For this review, take the finished solid that the model builds, in its own axes (mm). A direction names the side the tool comes from. Give positions to 0.01 mm unless a question says otherwise; leave off trailing zeros. Loops run counter-clockwise (first coordinate to the right, second up) from the corner with the lowest first, then second, coordinate; pieces in that order, holes last. Notation, with made-up numbers: (11, -9.75) - (17, -9.75) arc R19 ccw to (17, 15.25) - close; hole circle Ø3 at (-5, 30). An arc over 180 degrees is marked (long way). Use CSV: the item, a comma, the result in double quotes. Start each with the question number.
1. Wall thickness on line 1 (Z direction, x = -20, y = 57); line 2 (X direction, y = 56, z = -103); line 3 (Y direction, x = -9, z = -40): over which ranges is each line inside the solid? List them lowest first.
2. Mouldability with a two-part tool opening along Y and no side actions: class faces 1 (the flat face through (-20, 10, -22)), 2 (the cylindrical face through (-9.86, 99.915, -38.698)), 3 (the cylindrical face through (-34.93, 63.007, -39.406)), 4 (the flat face through (-20, 20, -40)) as pulls with the +Y half, pulls with the -Y half, needs draft (parallel to the pull), parting line crosses it, or undercut.
3. For faces 5 (the flat face through (-20, 54, -93)), 6 (the flat face through (-20, 10, -58)), 7 (the flat face through (-20, 82, -48)), 8 (the flat face through (-20, 64, -94)), list the 3-axis set-ups (+Z, -Z, +X, -X, +Y, -Y) from which the entire face can be reached by the end or side of a thin tool; tool diameter is ignored.
4. Take a section at D-D on z = -101.5. Give the boundary of the cut face in (x, y).
5. Take a section at B-B on z = -40. Give the boundary of the cut face in (x, y).
6. For pin 1 (11 mm diameter, centred on y = 61.5, z = 11.5, fed in from +X); pin 2 (22 mm diameter, centred on x = -27.5, y = 8.5, fed in from -Z); pin 3 (3 mm diameter, centred on x = -23.5, y = 87, fed in from +Z) (3 decimals); pin 4 (6 mm diameter, centred on x = -20, z = 23, fed in from +Y) (3 decimals), all flat-tipped, find the tip position at first contact; note any pin that passes through.
7. Take a section at A-A on y = 7.5. Give the boundary of the cut face in (x, z).
8. Take a section at C-C on x = -7. Give the boundary of the cut face in (y, z).
Autodesk Inventor part; units mm, degrees
ref_plane "YZ Plane" through (0, 0, 0) normal (1, 0, 0) x (0, 1, 0)
ref_plane "XZ Plane" through (0, 0, 0) normal (0, 1, 0) x (-1, 0, 0)
ref_plane "XY Plane" through (0, 0, 0) normal (0, 0, 1) x (1, 0, 0)
sketch "Sketch1" plane through (0, 0, 0) normal (1, 0, 0) x (0, 1, 0)
  line L0 (0, 0) -> (54, 0)
  line L1 (54, 0) -> (54, -80)
  line L2 (54, -80) -> (0, -80)
  line L3 (0, -80) -> (0, 0)
  dimension "d0" = 80
  dimension "d1" = 54
extrude "Extrusion1" add sketch "Sketch1" against normal blind 40
sketch "Sketch2" plane through (0, 0, 0) normal (1, 0, 0) x (0, 0, -1)
  line L0 (22, 20) -> (58, 20)
  line L1 (0, 0) -> (80, 0)
  line L2 (0, 54) -> (80, 54)
  line L3 (40, 54) -> (40, 0)
  line L4 (22, 20) -> (22, 0)
  line L5 (58, 20) -> (58, 0)
  line L6 (22, 0) -> (58, 0)
  line L7 (80, 0) -> (0, 0)
  point P0 (40, 20)
  dimension "d4" = 36
  dimension "d5" = 20
extrude "Extrusion2" cut sketch "Sketch2" against normal blind 40
sketch "Sketch3" plane through (0, 54, 0) normal (0, 1, 0) x (1, 0, 0)
  line L0 (-40, 58) -> (-40, 22)
  line L1 (-40, 40) -> (0, 40)
  line L2 (0, 22) -> (0, 58)
  line L3 (0, 0) -> (-40, 0)
  line L4 (-20, 0) -> (-20, 80) construction
  line L5 (0, 80) -> (-40, 80)
  circle A0 centre (-20, 103) radius 5
  arc A1 (-10, 103) -> (-30, 103) centre (-20, 103) ccw
  line L6 (-40, 40) -> (-40, 103)
  line L7 (-40, 103) -> (-30, 103)
  line L8 (0, 40) -> (0, 103)
  line L9 (0, 103) -> (-10, 103)
  circle A2 centre (-20, -23) radius 5
  arc A3 (-30, -23) -> (-10, -23) centre (-20, -23) ccw
  line L10 (-40, 40) -> (-40, -23)
  line L11 (-40, -23) -> (-30, -23)
  line L12 (0, 40) -> (0, -23)
  line L13 (0, -23) -> (-10, -23)
  line L14 (-10, 103) -> (-10, -23)
  line L15 (-30, 103) -> (-30, -23)
  point P0 (-10, 0)
  point P1 (-30, 0)
  point P2 (-30, 80)
  point P3 (-10, 80)
  dimension "d8" = 10
  dimension "d9" = 20
  dimension "d10" = 126
  dimension "d11" = 10
extrude "Extrusion3" add sketch "Sketch3" along normal blind 74
sketch "Sketch4" plane through (0, 0, 0) normal (1, 0, 0) x (0, 0, -1)
  line L0 (-4, 54) -> (84, 54)
  line L1 (-23, 128) -> (103, 128)
  line L2 (40, 128) -> (40, 0)
  line L3 (58, 0) -> (80, 0)
  line L4 (84, 54) -> (84, 59)
  circle A0 centre (40, 90) radius 19
  circle A1 centre (40, 90) radius 10
  circle A2 centre (40, 90) radius 27
  line L5 (5, 90) -> (75, 90)
  line L6 (5, 90) -> (-4, 54)
  line L7 (75, 90) -> (84, 54)
  line L8 (-23, 54) -> (-33, 54)
  line L9 (113, 54) -> (113, 128)
  line L10 (113, 54) -> (103, 54)
  line L11 (-33, 54) -> (113, 54)
  line L12 (-23, 128) -> (-33, 128)
  line L13 (-33, 128) -> (113, 128)
  line L14 (-33, 128) -> (-33, 54)
  line L15 (-33, 54) -> (-33, 128)
  line L16 (13, 90) -> (67, 90)
  line L17 (13, 90) -> (67, 90)
  point P0 (0, 0)
  point P1 (40, 54)
  point P2 (59, 90)
  point P3 (21, 90)
  point P4 (30, 90)
  point P5 (50, 90)
  dimension "d14" = 88
  dimension "d15" = 54
  dimension "d16" = 5
  dimension "d17" = 38
  dimension "d18" = 20
  dimension "d22" = 70
  dimension "d23" = 36
  dimension "d28" = 54
extrude "Extrusion4" cut sketch "Sketch4" against normal blind 74 contours L11 L8 L14 L12 L1 L2 A2 L5 L6 | L7 L5 A2 L2 L1 L13 L9 L10 L11
extrude "Extrusion5" cut sketch "Sketch4" against normal blind 74 contours A2 L5 A0 L2 | L2 A0 L5 A2 | A2 L2 A0 L5 | A0 L5 A1 L2 | L2 A1 L5 A0 | L5 A0 L2 A2 | A0 L2 A1 L5 | A1 L5 L2 | L2 L5 A1 | L5 A1 L2 A0 | A1 L2 L5 | L2 A1 L5
extrude "Extrusion6" add sketch "Sketch4" against normal blind 30 contours A2 L5 A0 L2 | L2 A0 L5 A2 picked at (15.8923, 87.9973) picked at (64.1077, 87.9973)
extrude "Extrusion7" add sketch "Sketch4" against normal blind 20 contours A0 L5 A1 L2 | L2 A1 L5 A0 picked at (24.1588, 88.5907) picked at (55.7576, 87.849)
extrude "Extrusion8" add sketch "Sketch4" against normal blind 20 contours A0 L2 A1 L5 | L5 A1 L2 A0 picked at (24.8696, 94.899) picked at (53.2638, 98.775)
extrude "Extrusion9" add sketch "Sketch3" along normal blind 10 contours L15 A1 L14 L5 | L3 L14 A3 L15
properties part number "Baitap3"
Check result:
1,line 1,"z = -113 to -108, -98 to 18, 28 to 33"
1,line 2,"x = -30 to -25, -15 to -10"
1,line 3,"y = 20 to 80, 100 to 109"
2,face 1,"needs draft"
2,face 2,"undercut"
2,face 3,"pulls with the +Y half"
2,face 4,"pulls with the -Y half"
3,face 5,"-Z, +X, -X, -Y"
3,face 6,"+X, -X, -Y"
3,face 7,"-X, +Y"
3,face 8,"-Z, +X, -X, +Y"
4,outline,"(-30, 54) - (-24.77, 54) - (-24.77, 64) - (-30, 64) - close; (-15.23, 54) - (-10, 54) - (-10, 64) - (-15.23, 64) - close"
5,outline,"(-40, 20) - (0, 20) - (0, 80) - (-20, 80) - (-20, 71) - (-30, 71) - (-30, 63) - (-40, 63) - close; (-20, 100) - (0, 100) - (0, 109) - (-20, 109) - close"
6,pin 1,"stops at x = -10"
6,pin 2,"stops at z = -80"
6,pin 3,"stops at z = -3.875"
6,pin 4,"passes through"
7,outline,"(-40, -80) - (0, -80) - (0, -58) - (-40, -58) - close; (-40, -22) - (0, -22) - (0, 0) - (-40, 0) - close"
8,outline,"(0, -80) - (54, -80) - (54, -84) - (90, -75) - (90, -59) arc R19 ccw to (90, -21) - (90, -5) - (54, 4) - (54, 0) - (0, 0) - (0, -22) - (20, -22) - (20, -58) - (0, -58) - close; hole circle Ø20 at (90, -40)"
